```python
from build123d import *

# Parameters (mm, degrees)
SKETCH7_W           = 60
SKETCH7_H           = 60
BOSS_EXTRUDE1_DEPTH = 30
SKETCH8_OUTSIDE_W   = 80
SKETCH8_OUTSIDE_H   = 80
CUT_EXTRUDE1_DEPTH  = 30
FILLET3_DEPTH       = 30
SKETCH6_W           = 60
SKETCH6_H           = 60
SKETCH6_R           = 2.25
BOSS_EXTRUDE2_DEPTH = 4
BOSS_EXTRUDE3_START = 34
SKETCH9_W           = 60
SKETCH9_H           = 60
SKETCH9_R           = 2.25
BOSS_EXTRUDE3_DEPTH = 4
SKETCH11_R          = 29
CUT_EXTRUDE3_DEPTH  = 50
FILLET4_R           = 2


with BuildPart() as part:
    # Sketch7 → Boss-Extrude1 (new body)
    with BuildSketch(Plane.XY):
        Rectangle(SKETCH7_W, SKETCH7_H)
    extrude(amount=BOSS_EXTRUDE1_DEPTH)

    # Sketch8 outside → Cut-Extrude1 (cut)
    with BuildSketch(Plane.XY.offset(30)):
        Rectangle(SKETCH8_OUTSIDE_W, SKETCH8_OUTSIDE_H)
        with BuildLine():
            Line((10, 30), (-10, 30))
            Line((-10, 30), (-10, 28.284271247))
            ThreePointArc((-10, 28.284271247), (-21.213203436, 21.213203436), (-28.284271247, 10))
            Line((-28.284271247, 10), (-30, 10))
            Line((-30, 10), (-30, -10))
            Line((-30, -10), (-28.284271247, -10))
            ThreePointArc((-28.284271247, -10), (-21.213203436, -21.213203436), (-10, -28.284271247))
            Line((-10, -28.284271247), (-10, -30))
            Line((-10, -30), (10, -30))
            Line((10, -30), (10, -28.284271247))
            ThreePointArc((10, -28.284271247), (21.213203436, -21.213203436), (28.284271247, -10))
            Line((28.284271247, -10), (30, -10))
            Line((30, -10), (30, 10))
            Line((30, 10), (28.284271247, 10))
            ThreePointArc((28.284271247, 10), (21.213203436, 21.213203436), (10, 28.284271247))
            Line((10, 28.284271247), (10, 30))
        make_face(mode=Mode.SUBTRACT)
    extrude(amount=-CUT_EXTRUDE1_DEPTH, mode=Mode.SUBTRACT)

    # Fillet3: read off the stored shape, not the designer's step
    # Fillet3 outline → Fillet3 (add)
    with BuildSketch(Plane.XY):
        with BuildLine():
            ThreePointArc((-28.284271247, 10), (-27.947444484, 10.905977573), (-27.581606794, 11.800634164))
            add(Edge.make_bspline(
                [(-27.581606794, 11.800634164), (-28.267504723, 10.197485832), (-30, 10)],
                knots=[0, 0, 0, 1, 1, 1], degree=2, weights=[1, 0.259369866, 1]))
            Line((-30, 10), (-28.284271247, 10))
        make_face()
        with BuildLine():
            add(Edge.make_bspline(
                [(-10, 30), (-10.197485832, 28.267504723), (-11.800634164, 27.581606794)],
                knots=[0, 0, 0, 1, 1, 1], degree=2, weights=[1, 0.259369866, 1]))
            ThreePointArc((-11.800634164, 27.581606794), (-10.905977573, 27.947444484), (-10, 28.284271247))
            Line((-10, 28.284271247), (-10, 30))
        make_face()
        with BuildLine():
            Line((-28.284271247, -10), (-30, -10))
            add(Edge.make_bspline(
                [(-30, -10), (-28.267504723, -10.197485832), (-27.581606794, -11.800634164)],
                knots=[0, 0, 0, 1, 1, 1], degree=2, weights=[1, 0.259369866, 1]))
            ThreePointArc((-27.581606794, -11.800634164), (-27.947444484, -10.905977573), (-28.284271247, -10))
        make_face()
        with BuildLine():
            ThreePointArc((-10, -28.284271247), (-10.905977573, -27.947444484), (-11.800634164, -27.581606794))
            add(Edge.make_bspline(
                [(-11.800634164, -27.581606794), (-10.197485832, -28.267504723), (-10, -30)],
                knots=[0, 0, 0, 1, 1, 1], degree=2, weights=[1, 0.259369866, 1]))
            Line((-10, -30), (-10, -28.284271247))
        make_face()
        with BuildLine():
            Line((10, -28.284271247), (10, -30))
            add(Edge.make_bspline(
                [(10, -30), (10.197485832, -28.267504723), (11.800634164, -27.581606794)],
                knots=[0, 0, 0, 1, 1, 1], degree=2, weights=[1, 0.259369866, 1]))
            ThreePointArc((11.800634164, -27.581606794), (10.905977573, -27.947444484), (10, -28.284271247))
        make_face()
        with BuildLine():
            ThreePointArc((28.284271247, -10), (27.947444484, -10.905977573), (27.581606794, -11.800634164))
            add(Edge.make_bspline(
                [(27.581606794, -11.800634164), (28.267504723, -10.197485832), (30, -10)],
                knots=[0, 0, 0, 1, 1, 1], degree=2, weights=[1, 0.259369866, 1]))
            Line((30, -10), (28.284271247, -10))
        make_face()
        with BuildLine():
            Line((28.284271247, 10), (30, 10))
            add(Edge.make_bspline(
                [(30, 10), (28.267504723, 10.197485832), (27.581606794, 11.800634164)],
                knots=[0, 0, 0, 1, 1, 1], degree=2, weights=[1, 0.259369866, 1]))
            ThreePointArc((27.581606794, 11.800634164), (27.947444484, 10.905977573), (28.284271247, 10))
        make_face()
        with BuildLine():
            ThreePointArc((10, 28.284271247), (10.905977573, 27.947444484), (11.800634164, 27.581606794))
            add(Edge.make_bspline(
                [(11.800634164, 27.581606794), (10.197485832, 28.267504723), (10, 30)],
                knots=[0, 0, 0, 1, 1, 1], degree=2, weights=[1, 0.259369866, 1]))
            Line((10, 30), (10, 28.284271247))
        make_face()
    extrude(amount=FILLET3_DEPTH)

    # Sketch6 → Boss-Extrude2 (add)
    with BuildSketch(Plane.XY):
        Rectangle(SKETCH6_W, SKETCH6_H)
        with Locations((25, 25)):
            Circle(SKETCH6_R, mode=Mode.SUBTRACT)
        with Locations(Location((-25, 25, 0), (0, 0, 180))):
            Circle(SKETCH6_R, mode=Mode.SUBTRACT)
        with Locations((-25, -25)):
            Circle(SKETCH6_R, mode=Mode.SUBTRACT)
        with Locations(Location((25, -25, 0), (0, 0, 180))):
            Circle(SKETCH6_R, mode=Mode.SUBTRACT)
    extrude(amount=-BOSS_EXTRUDE2_DEPTH)

    # Sketch9 → Boss-Extrude3 (add)
    with BuildSketch(Plane.XY.offset(BOSS_EXTRUDE3_START)):
        Rectangle(SKETCH9_W, SKETCH9_H)
        with Locations((25, 25)):
            Circle(SKETCH9_R, mode=Mode.SUBTRACT)
        with Locations(Location((-25, 25, 0), (0, 0, 180))):
            Circle(SKETCH9_R, mode=Mode.SUBTRACT)
        with Locations((-25, -25)):
            Circle(SKETCH9_R, mode=Mode.SUBTRACT)
        with Locations(Location((25, -25, 0), (0, 0, 180))):
            Circle(SKETCH9_R, mode=Mode.SUBTRACT)
    extrude(amount=-BOSS_EXTRUDE3_DEPTH)

    # Sketch11 → Cut-Extrude3 (cut)
    with BuildSketch(Plane.XY.offset(34)):
        Circle(SKETCH11_R)
    extrude(amount=-CUT_EXTRUDE3_DEPTH, mode=Mode.SUBTRACT)

    # Fillet4
    fillet4_edges = [part.edges().sort_by_distance(p)[0] for p in [
        (-30, -30, -2),
        (-30, -30, 32),
        (30, -30, 32),
        (30, -30, -2),
        (30, 30, -2),
        (30, 30, 32),
        (-30, 30, -2),
        (-30, 30, 32),
    ]]
    fillet(fillet4_edges, radius=FILLET4_R)


solid = part.part
```
Design review of the part built by this model. Coordinates are the model's own, in mm. A direction names the side the tool comes from. Coordinates: 2 decimals unless noted, no trailing zeros. Order: outer loops, then holes, each group sorted by start corner. A loop starts at its lowest first (then second) coordinate and runs counter-clockwise, first axis right, second up. Notation, with made-up numbers: (0.25, 8) - (49.25, 8) arc R16 ccw to (49.25, 13) - close; hole circle Ø3 at (35, -18.5). An arc over 180 degrees is marked (long way). Answer in a Markdown table with one row per item.
(1) Clearance check with flat-ended pins moving along their axes: pin 1 (7 mm diameter, centred on x = -25, y = 25, fed in from +Z); pin 2 (6 mm diameter, centred on x = 17.5, y = -19, fed in from +Z); pin 3 (3 mm diameter, centred on x = -23, z = 13.5, fed in from +Y); pin 4 (1 mm diameter, centred on y = 12, z = 23, fed in from +X). State where each tip first meets the part, or that it passes through.
Checked values:
| item | result |
|---|---|
| pin 1 | z = 34 |
| pin 2 | through |
| pin 3 | y = 20.92 |
| pin 4 | x = 27.81 |
(2) The part is to be moulded in two halves that separate along Y. For faces 4 (the cylindrical face through (-23.962, -26.996, 32.028)), 5 (the cylindrical face through (26.038, 23.004, 32.028)), 6 (the flat face through (0, 30, 15)), 7 (the flat face through (24, -22, 0)), say which applies: released by +Y, released by -Y, zero draft, split by the parting line, or undercut.
Checked values:
| item | result |
|---|---|
| face 4 | undercut |
| face 5 | undercut |
| face 6 | released by +Y |
| face 7 | zero draft |
(3) Consider section C-C on x = -16.5. State the section outline as (y, z) points.
Checked values:
| item | result |
|---|---|
| outline | (-30, -4) - (-23.85, -4) - (-23.85, 34) - (-30, 34) - (-30, 30) - (-25.05, 30) - (-25.05, 0) - (-30, 0) - close; (23.85, -4) - (30, -4) - (30, 0) - (25.05, 0) - (25.05, 30) - (30, 30) - (30, 34) - (23.85, 34) - close |
(4) For faces 1 (the cylindrical face through (21.1, -21.326, 15.21)), 2 (the flat face through (24, 22, 0)), 3 (the flat face through (-22, 22, 0)), list the 3-axis set-ups (+Z, -Z, +X, -X, +Y, -Y) from which the entire face can be reached by the end or side of a thin tool; tool diameter is ignored.
Checked values:
| item | result |
|---|---|
| face 1 | +X, -Y |
| face 2 | +X, +Y |
| face 3 | -X, +Y |
(5) Consider section B-B on x = 25. Give the number of separate pieces and of enclosed holes in the cut face, plus the area to 3 significant figures.
Checked values:
| item | result |
|---|---|
| separate pieces | 6 |
| enclosed holes | 0 |
| area | 286 mm^2 |
(6) Wall thickness on line 1 along Z through (x, y) = (18, 25.5); line 2 along Y through (x, z) = (0, 20); line 3 along Y through (x, z) = (25, 32): over which ranges is each line inside the solid? List them lowest first. Write a range as from..to.
Checked values:
| item | result |
|---|---|
| line 1 | -4..0, 30..34 |
| line 2 | -30..-29, 29..30 |
| line 3 | -30..-27.25, -22.75..-14.7, 14.7..22.75, 27.25..30 |
(7) Consider section A-A on y = 0. State the section outline as (x, z) points, plus the area to 3 significant figures.
Checked values:
| item | result |
|---|---|
| outline | (-30, -4) - (-29, -4) - (-29, 34) - (-30, 34) - close; (29, -4) - (30, -4) - (30, 34) - (29, 34) - close |
| area | 76.0 mm^2 |
